Can you work these out from the drawing? Everything is in mm from the part's minimum corner. Coordinates: 2 decimals unless noted, no trailing zeros. Loops run counter-clockwise (first coordinate to the right, second up) from the corner with the lowest first, then second, coordinate; pieces in that order, holes last.
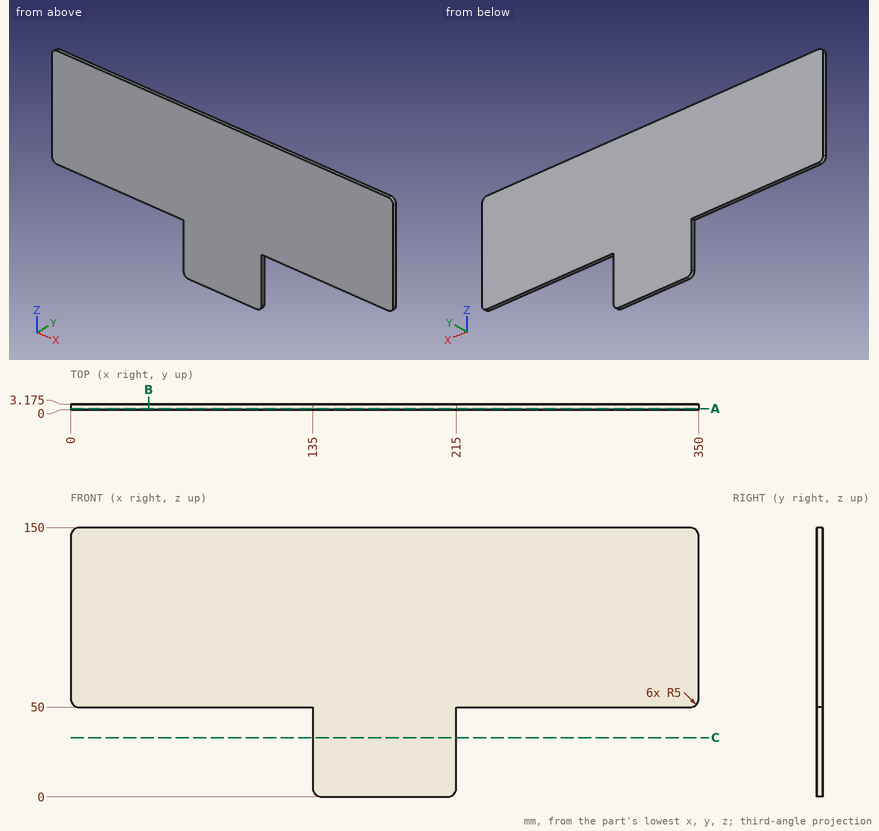
Item 1: Suppose I cut it at A-A, the plane y = 0.55. Please give me the cut outline in (x, z), plus the area to 3 significant figures.
Results are:
outline: (0, 55) arc R5 ccw to (5, 50) - (135, 50) - (135, 5) arc R5 ccw to (140, 0) - (210, 0) arc R5 ccw to (215, 5) - (215, 50) - (345, 50) arc R5 ccw to (350, 55) - (350, 145) arc R5 ccw to (345, 150) - (5, 150) arc R5 ccw to (0, 145) - close
area: 39,000 mm2
Item 2: I'm going to push flat-ended pins straight in: P1, Ø1.6, axis at y = 2.5, z = 20.5, coming from the -X side; P2, Ø1.6, axis at x = 283, y = 2, coming from the -Z side. Where does each tip first touch, or does it pass through?
Results are:
P1: stops at x = 135
P2: stops at z = 50
Item 3: Suppose I cut it at C-C, the plane z = 33. Please give me the cut outline in (x, y) (3 decimals), plus the area to 3 significant figures.
Results are:
outline: (135, 0) - (215, 0) - (215, 3.175) - (135, 3.175) - close
area: 254 mm2
Item 4: I need wall thicknesses on line 1 along Z through (x, y) = (72.5, 0.3); line 2 along X through (y, z) = (2.05, 46). Which ranges of each line are inside material? Lowest first, please.
Results are:
line 1: z = 50 to 150
line 2: x = 135 to 215
Item 5: Suppose I cut it at B-B, the plane x = 43.5. Please give me the cut outline in (y, z) (3 decimals).
Results are:
outline: (0, 50) - (3.175, 50) - (3.175, 150) - (0, 150) - close
